Part model, mm, in its own coordinate system. Round coordinates to 2 decimals unless told otherwise and drop trailing zeros. Order: outer loops, then holes, each group sorted by start corner. A loop starts at its lowest first (then second) coordinate and runs counter-clockwise, first axis right, second up. Notation, with made-up numbers: (47.5, 86.25) -> (103.5, 86.25) arc R11 cw to (103.5, 93.25) -> close; hole circle Ø10 at (-36, 23). An arc over 180 degrees is marked (long way). Answer as a JSON object with one key per item and string values. Group by question number.
```python
from build123d import *

# Parameters (mm, degrees)
F0_W           = 31.75
F0_H           = 38.1
F1_DEPTH       = 3.175
F3_D           = 4.4
F3_DEPTH       = 12.7
F3_CSINK_D     = 8.96
F3_CSINK_ANGLE = 90
F3_TIP         = 1.3218933619


with BuildPart() as f1:
    # F0 (on Front) → F1 (new body, symmetric)
    with BuildSketch(Plane.XZ):
        Rectangle(F0_W, F0_H)
    extrude(amount=F1_DEPTH, both=True)

    # F3
    with Locations(Plane.XZ.offset(3.175)):
        with Locations((0, 0), (0, -12.7)):
            CounterSinkHole(F3_D / 2, F3_CSINK_D / 2, depth=F3_DEPTH, counter_sink_angle=F3_CSINK_ANGLE)
            with Locations((0, 0, -(F3_DEPTH + F3_TIP / 2))):  # 118° drill point
                Cone(0, F3_D / 2, F3_TIP, mode=Mode.SUBTRACT)


solid = f1.part
```
Q1. Band-saw the part on D-D (y = -2.25). List the corners of the cut face in (x, z) (3 decimals).
Q2. Band-saw the part on B-B (z = -12.7). List the corners of the cut face in (x, y) (3 decimals), plus the area to 3 significant figures.
Q3. Two-plate mould, pull along Z, no slides. Class faces 1 (the flat face through (-15.875, 0, 0)), 2 (the flat face through (0, 0, -19.05)), 3 (the conical face through (1.834, -1.006, -1.406)): +Z half, -Z half, draft (parallel to the pull), parting line (faces both ways), or undercut.
Q4. Drop a flat-ended pin along its axis: pin 1 Ø5.5 at (x, z) = (0, 0) entering from -Y (3 decimals). Give the stop position or say it passes through.
Q5. Band-saw the part on C-C (y = 2.75). List the corners of the cut face in (x, z) (3 decimals).
Q6. Wall check: line 1 (Z direction, x = 0, y = 0.1); line 2 (X direction, y = 0.8, z = 0) (3 decimals); line 3 (Z direction, x = -0.5, y = 0.5). Give the ranges that are in metal, low to high. Write a range as [from, to].
Q7. Band-saw the part on A-A (x = 0). List the corners of the cut face in (y, z) (3 decimals), plus the area to 3 significant figures.
Completed:
{
 "1": {"outline": "(-15.875, -19.05) -> (15.875, -19.05) -> (15.875, 19.05) -> (-15.875, 19.05) -> close; hole circle Ø7.11 at (0, -12.7); hole circle Ø7.11 at (0, 0)"},
 "2": {"outline": "(-15.875, -3.175) -> (-4.48, -3.175) -> (-2.2, -0.895) -> (-2.2, 3.175) -> (-15.875, 3.175) -> close; (2.2, -0.895) -> (4.48, -3.175) -> (15.875, -3.175) -> (15.875, 3.175) -> (2.2, 3.175) -> close", "area": "168 mm2"},
 "3": {"face 1": "draft", "face 2": "-Z half", "face 3": "undercut"},
 "4": {"pin 1": "y = -1.445"},
 "5": {"outline": "(-15.875, -19.05) -> (15.875, -19.05) -> (15.875, 19.05) -> (-15.875, 19.05) -> close; hole circle Ø4.4 at (0, -12.7); hole circle Ø4.4 at (0, 0)"},
 "6": {"line 1": "[-19.05, -14.9], [-10.5, -2.2], [2.2, 19.05]", "line 2": "[-15.875, -2.2], [2.2, 15.875]", "line 3": "[-19.05, -14.84], [-10.56, -2.14], [2.14, 19.05]"},
 "7": {"outline": "(-3.175, -19.05) -> (3.175, -19.05) -> (3.175, -14.9) -> (-0.895, -14.9) -> (-3.175, -17.18) -> close; (-3.175, -8.22) -> (-0.895, -10.5) -> (3.175, -10.5) -> (3.175, -2.2) -> (-0.895, -2.2) -> (-3.175, -4.48) -> close; (-3.175, 4.48) -> (-0.895, 2.2) -> (3.175, 2.2) -> (3.175, 19.05) -> (-3.175, 19.05) -> close", "area": "176 mm2"}
}
